```python
from build123d import *

# Parameters (mm, degrees)
F1_DEPTH = 10


with BuildPart() as f1:
    # F0 (on Front) → F1 (new body)
    with BuildSketch(Plane.XZ):
        with BuildLine():
            ThreePointArc((-55, 38.75), (-58.661165, 47.588835), (-67.5, 51.25))
            ThreePointArc((-67.5, 51.25), (-76.338835, 29.911165), (-55, 38.75))
        make_face()
        Polygon((-135, 0), (0, 0), (0, 70), (-67.5, 77.5), (-135, 85), align=None)
        with BuildLine():
            ThreePointArc((-55, 38.75), (-76.338835, 29.911165), (-67.5, 51.25))
            ThreePointArc((-67.5, 51.25), (-58.661165, 47.588835), (-55, 38.75))
        make_face(mode=Mode.SUBTRACT)
    extrude(amount=F1_DEPTH)


solid = f1.part
```
The listing builds one solid part. Answer for the finished solid, in the listing's coordinates (mm). Coordinates: 2 decimals unless noted, no trailing zeros. Write each loop counter-clockwise with the first axis right and the second up, starting at its lowest first coordinate (ties: lowest second). Pieces come first, ordered by that corner, then holes. Notation, with made-up numbers: (81.5, -9.75) - (128.5, -9.75) arc R27 ccw to (128.5, 8.25) - close; hole circle Ø1 at (47.5, -18). An arc over 180 degrees is marked (long way). Return JSON: item names as keys, results as strings. Group by question number.
1. A cutting plane is placed at A-A, the plane y = -4.75. Determine the outline of the cut face in (x, z).
2. A cutting plane is placed at D-D, the plane x = -47. Determine the outline of the cut face in (y, z), plus the area to 3 significant figures.
3. A cutting plane is placed at B-B, the plane z = 33. Determine the outline of the cut face in (x, y), plus the area to 3 significant figures.
4. A cutting plane is placed at C-C, the plane x = -69. Determine the outline of the cut face in (y, z), plus the area to 3 significant figures.
5. Straight lines are drawn through the part: L1, parallel to X at y = -5.5, z = 38.75; L2, parallel to X at y = -1.5, z = 47.5; L3, parallel to Z at x = -67.5, y = -5.75. For each, find the intervals that lie inside material, in ascending order.
Ans:
{
 "1": {"outline": "(-135, 0) - (0, 0) - (0, 70) - (-135, 85) - close; hole circle Ø25 at (-67.5, 38.75)"},
 "2": {"outline": "(-10, 0) - (0, 0) - (0, 75.22) - (-10, 75.22) - close", "area": "752 mm²"},
 "3": {"outline": "(-135, -10) - (-78.6, -10) - (-78.6, 0) - (-135, 0) - close; (-56.4, -10) - (0, -10) - (0, 0) - (-56.4, 0) - close", "area": "1,130 mm²"},
 "4": {"outline": "(-10, 0) - (0, 0) - (0, 26.34) - (-10, 26.34) - close; (-10, 51.16) - (0, 51.16) - (0, 77.67) - (-10, 77.67) - close", "area": "528 mm²"},
 "5": {"L1": "-135 to -80, -55 to 0", "L2": "-135 to -76.43, -58.57 to 0", "L3": "0 to 26.25, 51.25 to 77.5"}
}
